Check sheet for the drawn part. Datum: minimum x, y, z corner. Units: mm. A direction names the side the tool comes from. Give positions to 0.01 mm unless a question says otherwise; leave off trailing zeros. Write each loop counter-clockwise with the first axis right and the second up, starting at its lowest first coordinate (ties: lowest second). Pieces come first, ordered by that corner, then holes. Notation, with made-up numbers: M 78.5,31 L 118.5,31 A16 ccw 118.5,53 Z; hole C 67.5,0.5 d2. An arc over 180 degrees is marked long. Write item = value, one per line. Start each with the question number.
1) Sectioned sample at D-D, the plane z = 18.5. Record the cut outline in (x, y), then the cut area to 3 significant figures.
2) Draft check along X on the marked faces 1, 2 and 3. Enter one of: pulls with the +X half, pulls with the -X half, needs draft (parallel to the pull), parting line crosses it, or undercut.
3) Gauge pin test, flat end, axial feed: pin 1 (3 mm diameter, centred on x = 21.5, z = 13, fed in from +Y). Record the tip position at first contact, or that the pin passes through.
4) Scan lines: L1, parallel to Y at x = 3, z = 20.4; L2, parallel to Z at x = 27, y = 18.25; L3, parallel to Y at x = 9, z = 13.5. Record each from-to range of solid material in increasing order.
5) Sectioned sample at B-B, the plane y = 7. Record the cut outline in (x, z).
6) Sectioned sample at A-A, the plane x = 27. Record the cut outline in (y, z), then the cut area to 3 significant figures.
7) Set-up check for the marked faces 4, 5 and 6: record each of +Z, -Z, +X, -X, +Y, -Y from which the full face is reachable in a straight line by a thin tool's end or side.
8) Sectioned sample at C-C, the plane y = 9. Count the separate pieces of the cut face and the enclosed holes in it, then the cut area to 3 significant figures.
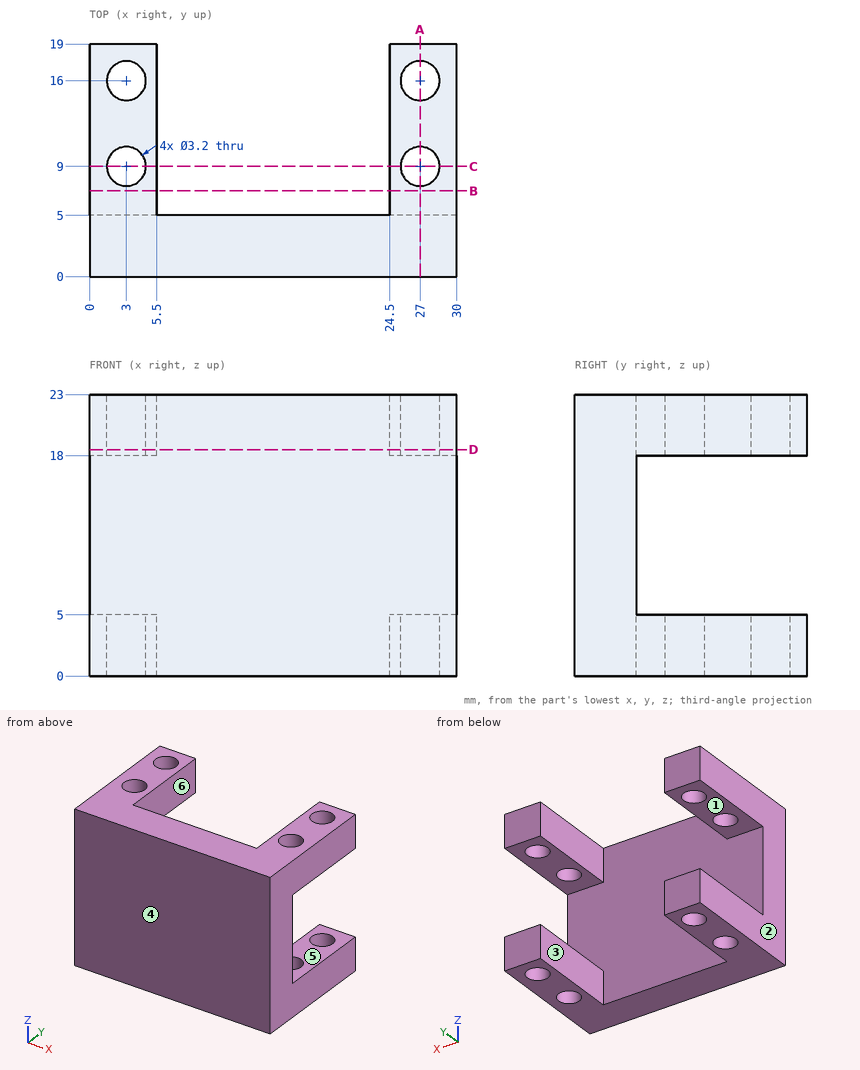
Data:
q1.outline = M 0,0 L 30,0 L 30,19 L 24.5,19 L 24.5,5 L 5.5,5 L 5.5,19 L 0,19 Z; hole C 3,9 d3.2; hole C 3,16 d3.2; hole C 27,9 d3.2; hole C 27,16 d3.2
q1.area = 272 mm2
q2.face_1 = needs draft
q2.face_2 = pulls with the -X half
q2.face_3 = undercut
q3.pin_1 = 5
q4.L1 = 0 to 7.4, 10.6 to 14.4, 17.6 to 19
q4.L2 = 0 to 5, 18 to 23
q4.L3 = 0 to 5
q5.outline = M 0,0 L 5.5,0 L 5.5,5 L 0,5 Z; M 0,18 L 5.5,18 L 5.5,23 L 0,23 Z; M 24.5,0 L 30,0 L 30,5 L 24.5,5 Z; M 24.5,18 L 30,18 L 30,23 L 24.5,23 Z
q6.outline = M 0,0 L 7.4,0 L 7.4,5 L 5,5 L 5,18 L 7.4,18 L 7.4,23 L 0,23 Z; M 10.6,0 L 14.4,0 L 14.4,5 L 10.6,5 Z; M 10.6,18 L 14.4,18 L 14.4,23 L 10.6,23 Z; M 17.6,0 L 19,0 L 19,5 L 17.6,5 Z; M 17.6,18 L 19,18 L 19,23 L 17.6,23 Z
q6.area = 191 mm2
q7.face_4 = +Z, -Z, +X, -X, -Y
q7.face_5 = +X, -X, +Y
q7.face_6 = +Z, -Z, +Y
q8.separate_pieces = 8
q8.enclosed_holes = 0
q8.area = 46.0 mm2
